Input: dimensioned drawing with shaded views. Units: mm. Origin: part minimum x, y, z. Round coordinates to 2 decimals unless told otherwise and drop trailing zeros. Loops run counter-clockwise (first coordinate to the right, second up) from the corner with the lowest first, then second, coordinate; pieces in that order, holes last.
1) Ray query, line 1 along Z through (x, y) = (23.5, 0.4); line 2 along X through (y, z) = (0.45, 31.09); line 3 along Z through (x, y) = (22, 0.25). Return the intervals inside material, ascending.
2) Section D-D, the plane y = 0.2. Return loops of the section in (x, z), and give its area (3 significant figures).
3) Section B-B, the plane z = 31.09. Return loops of the section in (x, y).
4) Section C-C, the plane z = 38.68. Return loops of the section in (x, y).
5) Section A-A, the plane x = 23.5. Return loops of the section in (y, z).
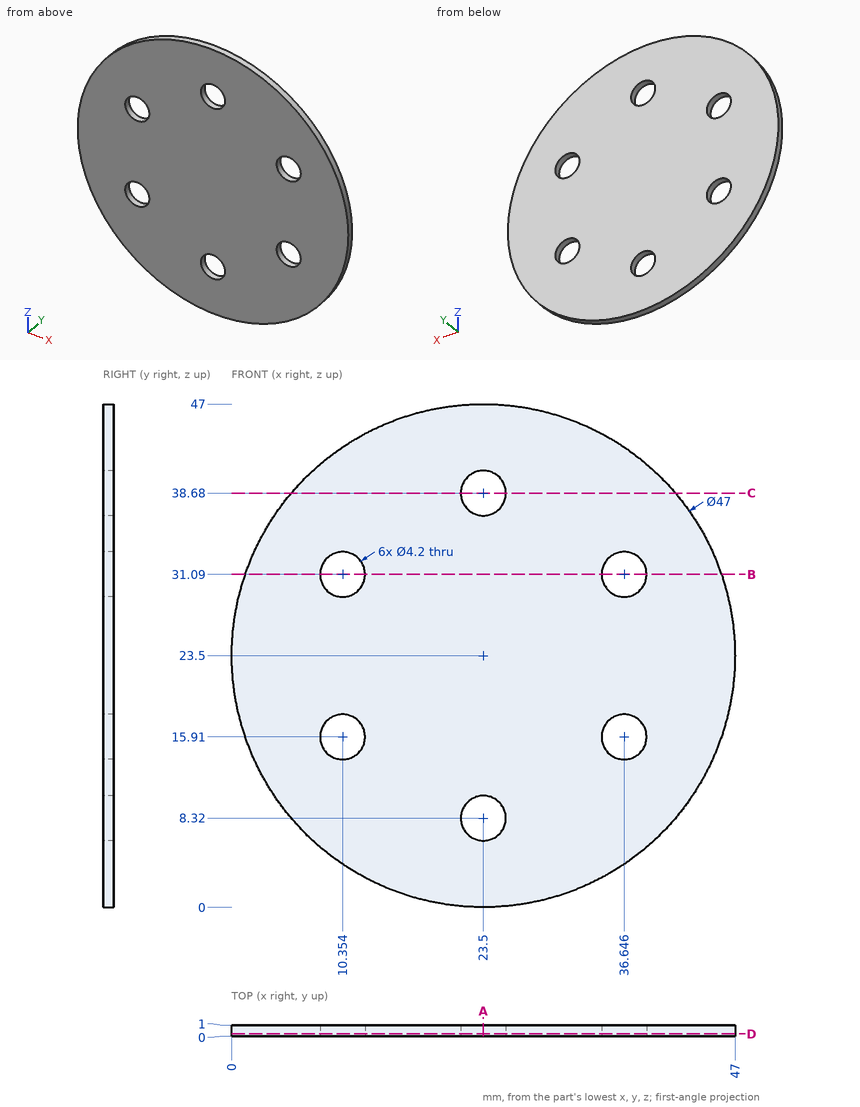
Final values:
1. line 1: z = 0 to 6.22, 10.42 to 36.58, 40.78 to 47
1. line 2: x = 1.26 to 8.25, 12.45 to 34.55, 38.75 to 45.74
1. line 3: z = 0.05 to 6.85, 9.79 to 37.21, 40.15 to 46.95
2. outline: circle Ø47 at (23.5, 23.5); hole circle Ø4.2 at (10.35, 15.91); hole circle Ø4.2 at (10.35, 31.09); hole circle Ø4.2 at (23.5, 8.32); hole circle Ø4.2 at (23.5, 38.68); hole circle Ø4.2 at (36.65, 15.91); hole circle Ø4.2 at (36.65, 31.09)
2. area: 1,650 mm2
3. outline: (1.26, 0) - (8.25, 0) - (8.25, 1) - (1.26, 1) - close; (12.45, 0) - (34.55, 0) - (34.55, 1) - (12.45, 1) - close; (38.75, 0) - (45.74, 0) - (45.74, 1) - (38.75, 1) - close
4. outline: (5.56, 0) - (21.4, 0) - (21.4, 1) - (5.56, 1) - close; (25.6, 0) - (41.44, 0) - (41.44, 1) - (25.6, 1) - close
5. outline: (0, 0) - (1, 0) - (1, 6.22) - (0, 6.22) - close; (0, 10.42) - (1, 10.42) - (1, 36.58) - (0, 36.58) - close; (0, 40.78) - (1, 40.78) - (1, 47) - (0, 47) - close
